from build123d import *

# Parameters (mm, degrees)
SKETCH2_W           = 250
SKETCH2_H           = 150
BOSS_EXTRUDE1_DEPTH = 10
SKETCH3_R           = 2
SKETCH3_W           = 50
SKETCH3_H           = 32
CUT_EXTRUDE1_DEPTH  = 10
SKETCH4_W           = 28
SKETCH4_H           = 15.597165116
CUT_EXTRUDE2_DEPTH  = 10
SKETCH5_R           = 1.5
SKETCH5_R_2         = 1.1
CUT_EXTRUDE3_DEPTH  = 147.116391962


with BuildPart() as part:
    # Sketch2 → Boss-Extrude1 (new body)
    with BuildSketch(Plane(origin=(0, 0, 0), x_dir=(1, 0, 0), z_dir=(0, 1, 0))):
        Rectangle(SKETCH2_W, SKETCH2_H)
    extrude(amount=BOSS_EXTRUDE1_DEPTH)

    # Sketch3 → Cut-Extrude1 (cut)
    with BuildSketch(Plane(origin=(0, 10, 0), x_dir=(1, 0, 0), z_dir=(0, 1, 0))):
        with Locations(Location((35, -13, 0), (0, 0, 270))):
            Circle(SKETCH3_R)
        with Locations(Location((75, -13, 0), (0, 0, 270))):
            Circle(SKETCH3_R)
        with Locations(Location((35, -65, 0), (0, 0, 270))):
            Circle(SKETCH3_R)
        with Locations(Location((75, -65, 0), (0, 0, 270))):
            Circle(SKETCH3_R)
        with Locations((55, -39)):
            Rectangle(SKETCH3_W, SKETCH3_H)
    extrude(amount=-CUT_EXTRUDE1_DEPTH, mode=Mode.SUBTRACT)

    # Sketch4 → Cut-Extrude2 (cut)
    with BuildSketch(Plane(origin=(0, 10, 0), x_dir=(1, 0, 0), z_dir=(0, 1, 0))):
        with Locations((-35.9, -10.201417442)):
            Rectangle(SKETCH4_W, SKETCH4_H)
    extrude(amount=-CUT_EXTRUDE2_DEPTH, mode=Mode.SUBTRACT)

    # Sketch5 → Cut-Extrude3 (cut, through all)
    with BuildSketch(Plane(origin=(0, 10, 0), x_dir=(1, 0, 0), z_dir=(0, 1, 0))):
        with Locations(Location((-10, -11.5, 0), (0, 0, 270))):
            Circle(SKETCH5_R)
        with Locations(Location((-57.5, -11.5, 0), (0, 0, 270))):
            Circle(SKETCH5_R)
        with Locations(Location((-19.3, -11.05, 0), (0, 0, 270))):
            Circle(SKETCH5_R_2)
    extrude(amount=-CUT_EXTRUDE3_DEPTH, mode=Mode.SUBTRACT)


solid = part.part
The listing builds one solid part. Answer for the finished solid, in the listing's coordinates (mm). A direction names the side the tool comes from. Round coordinates to 2 decimals unless told otherwise and drop trailing zeros. Order: outer loops, then holes, each group sorted by start corner. A loop starts at its lowest first (then second) coordinate and runs counter-clockwise, first axis right, second up. Notation, with made-up numbers: (46, -33.5) -> (97, -33.5) arc R13 ccw to (97, -19.5) -> close; hole circle Ø11 at (87.5, -6). An arc over 180 degrees is marked (long way). One line per item, written item: value.
Item 1: Given P1, Ø3, axis at x = 75, z = 13, coming from the +Y side, flat-ended and moving along its own axis, determine where the tip first touches the part or whether it passes through.
Taken from the geometry:
P1: passes through
Item 2: For faces 1 (the flat face through (-2, 10, -1)), 2 (the flat face through (55, 5, 55)), determine the directions among +Z, -Z, +X, -X, +Y, -Y from which every point of the face is accessible in a straight line to the end or side of a thin tool.
Taken from the geometry:
face 1: +Z, -Z, +X, -X, +Y
face 2: +Y, -Y
Item 3: For a pull along Z with two mould halves and no side action, classify faces 3 (the flat face through (-36, 5, 18)), 4 (the flat face through (-2, 5, -75)), 5 (the flat face through (-2, 0, -1)) as released by +Z, released by -Z, zero draft, split by the parting line, or undercut.
Taken from the geometry:
face 3: undercut
face 4: released by -Z
face 5: zero draft
Item 4: Straight lines are drawn through the part: L1, parallel to X at y = 7, z = 65; L2, parallel to X at y = 5.25, z = 52.5; L3, parallel to Z at x = -56.5, y = 7. For each, find the intervals that lie inside material, in ascending order.
Taken from the geometry:
L1: x = -125 to 33, 37 to 73, 77 to 125
L2: x = -125 to 30, 80 to 125
L3: z = -75 to 10.38, 12.62 to 75
Item 5: Find section C-C, the plane y = 8.5. State how many separate pieces and enclosed holes the cut face has, then the cut area to 3 significant figures.
Taken from the geometry:
separate pieces: 1
enclosed holes: 9
area: 35,400 mm2
Item 6: Find section B-B, the plane z = 50.5. Give the vertices of the cut face in (x, y).
Taken from the geometry:
outline: (-125, 0) -> (30, 0) -> (30, 10) -> (-125, 10) -> close; (80, 0) -> (125, 0) -> (125, 10) -> (80, 10) -> close
Item 7: Find section A-A, the plane x = 55. Give the vertices of the cut face in (y, z).
Taken from the geometry:
outline: (0, -75) -> (10, -75) -> (10, 23) -> (0, 23) -> close; (0, 55) -> (10, 55) -> (10, 75) -> (0, 75) -> close
